Geometry check sheet. Reference: the model listing, model coordinates, mm. Give positions to 0.01 mm unless a question says otherwise; leave off trailing zeros. Loops run counter-clockwise (first coordinate to the right, second up) from the corner with the lowest first, then second, coordinate; pieces in that order, holes last.
```python
from build123d import *

# Parameters (mm, degrees)
SKETCH1_W           = 12.394273752
SKETCH1_H           = 12.46455313
BOSS_EXTRUDE1_DEPTH = 65
CUT_EXTRUDE1_START  = -12.394274
SKETCH2_R           = 2.75
CUT_EXTRUDE1_DEPTH  = 12.394274


with BuildPart() as part:
    # Sketch1 → Boss-Extrude1 (new body)
    with BuildSketch(Plane.XY):
        with Locations((-36.202863124, 114.417723435)):
            Rectangle(SKETCH1_W, SKETCH1_H)
    extrude(amount=-BOSS_EXTRUDE1_DEPTH)

    # Sketch2 → Cut-Extrude1 (cut)
    with BuildSketch(Plane.ZY.offset(42.4).offset(CUT_EXTRUDE1_START)):
        with Locations(Location((-52.5, 114.417723435, 0), (0, 0, 180))):
            Circle(SKETCH2_R)
        with Locations(Location((-12.5, 114.417723435, 0), (0, 0, 180))):
            Circle(SKETCH2_R)
    extrude(amount=CUT_EXTRUDE1_DEPTH, mode=Mode.SUBTRACT)


solid = part.part
```
1) Scan lines: line 1 along Z through (x, y) = (-32, 115); line 2 along Y through (x, z) = (-36.25, -52.5); line 3 along Z through (x, y) = (-41.5, 116.5). Record each from-to range of solid material in increasing order.
2) Mould release check, pull along Z, two halves, no side actions. Record for faces 1 (the flat face through (-36, 115, -65)), 2 (the cylindrical face through (-36.1, 117.1, -11.9)), 3 (the flat face through (-36, 115, 0)), 4 (the flat face through (-36, 120.65, -32)): +Z half, -Z half, draft (parallel to the pull), parting line (faces both ways), or undercut.
3) Sectioned sample at B-B on x = -37. Enter the section's corners in (y, z).
4) Sectioned sample at A-A on z = -52.5. Enter the section's corners in (x, y), plus the area to 3 significant figures.
Determined:
1. line 1: z = -65 to -55.19, -49.81 to -15.19, -9.81 to 0
1. line 2: y = 108.19 to 111.67, 117.17 to 120.65
1. line 3: z = -65 to -54.3, -50.7 to -14.3, -10.7 to 0
2. face 1: -Z half
2. face 2: undercut
2. face 3: +Z half
2. face 4: draft
3. outline: (108.19, -65) - (120.65, -65) - (120.65, 0) - (108.19, 0) - close; hole circle Ø5.5 at (114.42, -52.5); hole circle Ø5.5 at (114.42, -12.5)
4. outline: (-42.4, 108.19) - (-30.01, 108.19) - (-30.01, 111.67) - (-42.4, 111.67) - close; (-42.4, 117.17) - (-30.01, 117.17) - (-30.01, 120.65) - (-42.4, 120.65) - close
4. area: 86.3 mm2
